Geometry: final body of the model. Coordinates: model frame, mm. Give positions to 0.01 mm unless a question says otherwise; leave off trailing zeros. Loops run counter-clockwise (first coordinate to the right, second up) from the corner with the lowest first, then second, coordinate; pieces in that order, holes last. Notation, with made-up numbers: M 53.25,82 L 67.25,82 A30 ccw 67.25,118 Z; hole C 34.5,-29 d5. An arc over 180 degrees is marked long. Put each result on its own line as item: value.
```python
from build123d import *

# Parameters (mm, degrees)
SKETCH1_R           = 72.401096357
SKETCH1_R_2         = 53.117079775
BOSS_EXTRUDE1_DEPTH = 20
FILLET8_R           = 10
FILLET9_R           = 10
FILLET10_R          = 10


with BuildPart() as part:
    # Sketch1 → Boss-Extrude1 (new body)
    with BuildSketch(Plane.XY):
        Circle(SKETCH1_R)
        Circle(SKETCH1_R_2, mode=Mode.SUBTRACT)
    extrude(amount=BOSS_EXTRUDE1_DEPTH)

    # Fillet8
    fillet8_edges = [part.edges().sort_by_distance(p)[0] for p in [
        (-53.117079775, 0, 20),
    ]]
    fillet(fillet8_edges, radius=FILLET8_R)

    # Fillet9
    # the kernel refuses this fillet: 10 mm, written as the material it takes off along each edge
    with BuildSketch(Plane(origin=(0, 0, 20), x_dir=(1, 0, 0), z_dir=(0, -1, 0))) as fillet9_piece_1:
        with BuildLine():
            CenterArc((62.401096357, -9.974335454), FILLET9_R, 0, 85.894204151)
            Line((72.401096357, -9.974335454), (72.601096357, -9.974335454))
            Line((72.601096357, -9.974335454), (72.601096357, 0))
            Line((72.601096357, 0), (72.401096357, 0.2))
            ThreePointArc((72.401096357, 0.2), (67.759088066, 0.2), (63.131399443, 0.199486709))
            Line((63.131399443, 0.199486709), (63.117079775, 0))
        make_face()
    revolve(axis=Axis((0, 0, 20), (0, 0, 1)), mode=Mode.SUBTRACT)

    # Fillet10
    fillet10_edges = [part.edges().sort_by_distance(p)[0] for p in [
        (-72.401096357, 0, 0),
    ]]
    fillet(fillet10_edges, radius=FILLET10_R)


solid = part.part
```
Item 1: Mould query, pull axis Y, two halves, no side actions, for faces 1 (the cylindrical face through (49.07, -20.34, 4.93)), 2 (the flat face through (46, 28, 0)). Classes: pulls with the +Y half, pulls with the -Y half, needs draft (parallel to the pull), parting line crosses it, or undercut.
Output values:
face 1: undercut
face 2: needs draft
Item 2: Section C-C on z = 6.25. Output: boundary loops of the cut face in (x, y).
Output values:
outline: C 0,0 d143.34; hole C 0,0 d106.23
Item 3: Line query: probe 1 along Y at (x, z) = (-13.5, 2.5); probe 2 along X at (y, z) = (20.5, 9); probe 3 along Y at (x, z) = (0, 7). Output: solid intervals per line, ascending. Write a range as [from, to].
Output values:
probe 1: [-67.68, -51.37], [51.37, 67.68]
probe 2: [-69.39, -49], [49, 69.39]
probe 3: [-71.94, -53.12], [53.12, 71.94]
Item 4: Pin query (flat end, axial travel): pin 1 Ø5 at (x, y) = (54.5, -51.5) entering from -Z; pin 2 Ø4 at (x, y) = (-57, 18.5) entering from +Z; pin 3 Ø12 at (x, z) = (49.5, 17.5) entering from -Y; pin 4 Ø3 at (x, z) = (-17.5, 14.5) entering from -Y. Return the tip coordinate at first contact, or that it passes through.
Output values:
pin 1: through
pin 2: z = 19.93
pin 3: y = -55.96
pin 4: y = -69.91
